Check sheet for the modelled part. Datum: model origin and axes. Units: mm. A direction names the side the tool comes from. Coordinates: 2 decimals unless noted, no trailing zeros. Loops run counter-clockwise (first coordinate to the right, second up) from the corner with the lowest first, then second, coordinate; pieces in that order, holes last. Notation, with made-up numbers: M -25.75,-21.5 L 19.25,-21.5 A16 cw 19.25,-0.5 Z; hole C 70.5,-4 d6. An arc over 180 degrees is marked long. Write each question's results on one line, items separated by ' | '. Start each with the question number.
from build123d import *

# Parameters (mm, degrees)
BOSS_EXTRUDE2_DEPTH      = 10
BOSS_EXTRUDE2_DEPTH_BACK = 10
CUT_EXTRUDE1_DEPTH       = 6
CUT_EXTRUDE1_DEPTH_BACK  = 6
SKETCH3_R                = 12


with BuildPart() as part:
    # Sketch1 → Boss-Extrude2 (new, two sides: drawn at the far end of the back side and taken through both)
    with BuildSketch(Plane.XY.offset(-BOSS_EXTRUDE2_DEPTH_BACK)):
        with BuildLine():
            ThreePointArc((10.908712115, 5), (-12, 0), (10.908712115, -5))
            Line((10.908712115, -5), (15.198684154, -5))
            ThreePointArc((15.198684154, -5), (16, 0), (15.198684154, 5))
            Line((15.198684154, 5), (10.908712115, 5))
        make_face()
        with BuildLine():
            Line((-4.898979486, 5), (4.898979486, 5))
            ThreePointArc((4.898979486, 5), (7, 0), (4.898979486, -5))
            Line((4.898979486, -5), (-4.898979486, -5))
            ThreePointArc((-4.898979486, -5), (-7, 0), (-4.898979486, 5))
        make_face(mode=Mode.SUBTRACT)
    extrude(amount=BOSS_EXTRUDE2_DEPTH + BOSS_EXTRUDE2_DEPTH_BACK)

    # Sketch3 → Cut-Extrude1 (cut, two sides: drawn at the far end of the back side and taken through both)
    with BuildSketch(Plane.XY.offset(-CUT_EXTRUDE1_DEPTH_BACK)):
        Circle(SKETCH3_R)
    extrude(amount=CUT_EXTRUDE1_DEPTH + CUT_EXTRUDE1_DEPTH_BACK, mode=Mode.SUBTRACT)


solid = part.part
Item 1: Section check C-C (y = 9). Record the cut outline in (x, z).
Item 2: Tool access check on faces 1 (the face through (1.8, -5.2, -10)), 2 (the face through (0, -5, 8)), 3 (the face through (13, 5, 0)), 4 (the face through (13, -5, 0)), 5 (the face through (12, 0, 0)). Record the directions out of +Z, -Z, +X, -X, +Y, -Y that give a thin tool (end or side, any length) a straight path to the whole face; none if there is none.
Item 3: Section check A-A (x = 0). Record the cut outline in (y, z), plus the area to 3 significant figures.
Item 4: Release check for a two-part mould opening along Y. For faces 6 (the face through (1.8, -5.2, 10)), 7 (the face through (16, 0, 0)), 8 (the face through (0, 5, 8)), 9 (the face through (-7, 0, 8)) record: +Y half, -Y half, draft (parallel to the pull), parting line (faces both ways), or undercut.
Item 5: Section check D-D (x = -9.5). Record the cut outline in (y, z), plus the area to 3 significant figures.
Item 6: Thickness scan on line 1 (Z direction, x = -4.5, y = 10); line 2 (X direction, y = -2.75, z = -8.75); line 3 (X direction, y = -1.5, z = 8.75). Record the ranges inside material, lowest first.
Item 7: Section check B-B (y = 0). Record the cut outline in (x, z).
Item 8: Depth check by flat-ended pin: P1, Ø5, axis at y = -3, z = -8, coming from the +X side; P2, Ø3, axis at y = 0.5, z = 0.5, coming from the -X side; P3, Ø1.2, axis at x = -1, z = -8, coming from the -Y side. Enter the tip coordinate at first touch or a pass-through.
Computed values:
1) outline: M -7.94,-10 L 7.94,-10 L 7.94,-6 L -7.94,-6 Z; M -7.94,6 L 7.94,6 L 7.94,10 L -7.94,10 Z
2) face 1: -Z, +X, -X, +Y, -Y | face 2: +Z, -Z | face 3: +Z, -Z, +X, +Y | face 4: +Z, -Z, +X, -Y | face 5: -X
3) outline: M -12,-10 L -5,-10 L -5,-6 L -12,-6 Z; M -12,6 L -5,6 L -5,10 L -12,10 Z; M 5,-10 L 12,-10 L 12,-6 L 5,-6 Z; M 5,6 L 12,6 L 12,10 L 5,10 Z | area: 112 mm²
4) face 6: draft | face 7: parting line | face 8: undercut | face 9: undercut
5) outline: M -7.33,-10 L 7.33,-10 L 7.33,-6 L -7.33,-6 Z; M -7.33,6 L 7.33,6 L 7.33,10 L -7.33,10 Z | area: 117 mm²
6) line 1: z = -10 to -6, 6 to 10 | line 2: x = -11.68 to -6.44, 6.44 to 15.76 | line 3: x = -11.91 to -6.84, 6.84 to 15.93
7) outline: M -12,-10 L -7,-10 L -7,-6 L -12,-6 Z; M -12,6 L -7,6 L -7,10 L -12,10 Z; M 7,-10 L 16,-10 L 16,10 L 7,10 L 7,6 L 12,6 L 12,-6 L 7,-6 Z
8) P1: stops at x = 15.99 | P2: stops at x = 11.83 | P3: stops at y = -11.99
